Build history of the part. All positions in model axes, mm. Give positions to 0.01 mm unless a question says otherwise; leave off trailing zeros. Order: outer loops, then holes, each group sorted by start corner. A loop starts at its lowest first (then second) coordinate and runs counter-clockwise, first axis right, second up. Notation, with made-up numbers: (22, -22) - (50, -22) arc R14 cw to (50, -18) - close; hole circle Ø10 at (74.5, -28.5). An arc over 180 degrees is marked (long way). Answer in a Markdown table with one row per item.
Autodesk Inventor part; units mm, degrees
ref_plane "YZ Plane" through (0, 0, 0) normal (1, 0, 0) x (0, 1, 0)
ref_plane "XZ Plane" through (0, 0, 0) normal (0, 1, 0) x (-1, 0, 0)
ref_plane "XY Plane" through (0, 0, 0) normal (0, 0, 1) x (1, 0, 0)
sketch "Sketch1" plane through (0, 0, 0) normal (1, 0, 0) x (0, 1, 0)
  line L0 (-172.4, 268.6) -> (172.4, 268.6)
  line L1 (172.4, 268.6) -> (172.4, -268.6)
  line L2 (172.4, -268.6) -> (-172.4, -268.6)
  line L3 (-172.4, -268.6) -> (-172.4, 268.6)
  point P0 (0, 0)
  dimension "d0" = 537.2
  dimension "d1" = 344.8
  dimension "d96" = 268.6
  dimension "d97" = 172.4
extrude "Extrusion1" add sketch "Sketch1" along normal blind 6.35
sketch "Sketch2" plane through (6.35, 0, 0) normal (1, 0, 0) x (0, 0, -1)
  circle A0 centre (-0.005, -43.5) radius 50.8
  line L0 (-268.6, 172.4) -> (-268.6, -172.4)
  line L1 (268.6, -172.4) -> (268.6, 172.4)
  line L2 (268.6, 172.4) -> (-268.6, 172.4)
  line L3 (-268.6, -172.4) -> (268.6, -172.4)
  dimension "d6" = 101.6
  dimension "d51" = 268.605
  dimension "d65" = 215.9
extrude "Extrusion2" cut sketch "Sketch2" against normal through all contours A0
sketch "Sketch5" plane through (6.35, 0, 0) normal (1, 0, 0) x (0, 0, -1)
  line L0 (-101.6, -43.5) -> (101.6, -43.5) construction
  circle A0 centre (-0.005, -43.5) radius 37.8815 construction
  circle A1 centre (-0.005, -43.5) radius 50.8
  point P0 (0, 0)
  dimension "d62" = 203.2
  dimension "d63" = 101.6
  dimension "d64" = 75.7631
hole "Hole1" at (6.35, -43.5, 101.6) at (6.35, -43.5, -101.6) direction (-1, 0, 0) diameter 7.1374 end through all
sketch "Sketch6" plane through (6.35, 0, 0) normal (1, 0, 0) x (0, 0, -1)
  line L0 (-88.9, 32.7) -> (88.9, 32.7) construction
  circle A0 centre (-0.005, -43.5) radius 50.8
  point P0 (0, 0)
  dimension "d73" = 177.8
  dimension "d75" = 88.9
  dimension "d76" = 76.2
hole "Hole2" at (6.35, 32.7, 88.9) at (6.35, 32.7, -88.9) direction (-1, 0, 0) diameter 6.7564 end through all
sketch "Sketch7" plane through (6.35, 0, 0) normal (1, 0, 0) x (0, 0, -1)
  line L0 (268.6, 172.4) -> (-268.6, 172.4)
  line L1 (-268.6, 172.4) -> (-268.6, -172.4)
  line L2 (-268.6, -172.4) -> (268.6, -172.4)
  point P0 (0, 0)
  point P1 (-248.6, 152.4)
  point P2 (-248.6, 101.6)
  point P3 (-197.8, 152.4)
  point P4 (-147, 152.4)
  point P5 (-248.6, 50.8)
  point P6 (-248.6, -50.8)
  point P7 (-248.6, -101.6)
  point P8 (-248.6, -152.4)
  point P9 (-197.8, -152.4)
  point P10 (-147, -152.4)
  dimension "d84" = 20
  dimension "d85" = 20
  dimension "d86" = 50.8
  dimension "d87" = 50.8
  dimension "d88" = 50.8
  dimension "d89" = 50.8
  dimension "d90" = 20
  dimension "d91" = 20
  dimension "d92" = 50.8
  dimension "d93" = 50.8
  dimension "d94" = 50.8
  dimension "d95" = 50.8
hole "Hole3" at (6.35, 152.4, 248.6) at (6.35, 101.6, 248.6) at (6.35, 152.4, 197.8) at (6.35, 152.4, 147) at (6.35, 50.8, 248.6) at (6.35, -50.8, 248.6) at (6.35, -101.6, 248.6) at (6.35, -152.4, 248.6) at (6.35, -152.4, 197.8) at (6.35, -152.4, 147) direction (-1, 0, 0) diameter 8.9916 end through all
mirror "Mirror1" about plane through (0, 0, 0) normal (0, 0, 1) of "Hole3"
properties part number "ODSY-0007-001" material "Aluminum 6061"
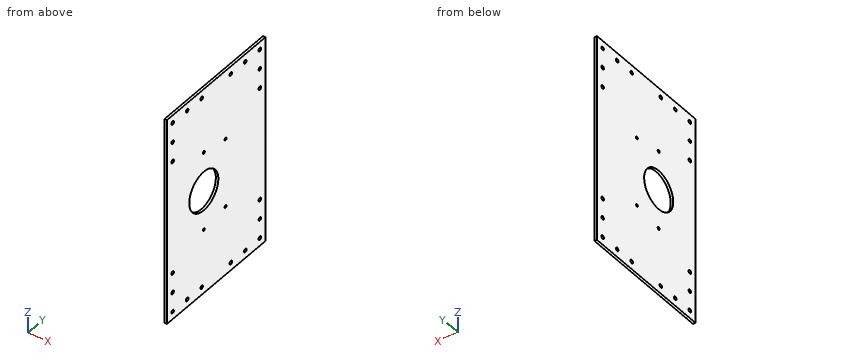
1. Probe line 1 (Z direction, x = 5.25, y = 101.6); line 2 (Y direction, x = 4.5, z = 147); line 3 (Y direction, x = 1.75, z = 146). List the from-to ranges inside material, lowest first.
Check result:
| item | result |
|---|---|
| line 1 | z = -268.6 to -253.1, -244.1 to 244.1, 253.1 to 268.6 |
| line 2 | y = -172.4 to -156.9, -147.9 to 147.9, 156.9 to 172.4 |
| line 3 | y = -172.4 to -156.78, -148.02 to 148.02, 156.78 to 172.4 |
2. Cut at B-B on z = -21. Write the cut outline in (x, y).
Check result:
| item | result |
|---|---|
| outline | (0, -172.4) - (6.35, -172.4) - (6.35, -89.75) - (0, -89.75) - close; (0, 2.75) - (6.35, 2.75) - (6.35, 172.4) - (0, 172.4) - close |
3. Cut at A-A on x = 5. Count the separate pieces of the cut face and the enclosed holes in it, and give its area (3 significant figures).
Check result:
| item | result |
|---|---|
| separate pieces | 1 |
| enclosed holes | 25 |
| area | 176,000 mm² |
